```python
from build123d import *

# Parameters (mm, degrees)
BOSS_EXTRUDE1_DEPTH  = 557.5
SKETCH2_W            = 37.5
SKETCH2_H            = 40
BOSS_EXTRUDE2_DEPTH  = 340
BOSS_EXTRUDE3_DEPTH  = 1115
SKETCH4_W            = 120
SKETCH4_H            = 22
CUT_EXTRUDE1_DEPTH   = 754.951092578
FILLET1_R            = 6
SKETCH8_W            = 20
SKETCH8_H            = 10
CUT_EXTRUDE3_DEPTH   = 754.951092578
SKETCH9_W            = 25
SKETCH9_H            = 25
SKETCH9_R            = 5.25
BOSS_EXTRUDE6_DEPTH  = 20
CHAMFER1_SIZE        = 4
SKETCH10_W           = 1014
SKETCH10_H           = 110
BOSS_EXTRUDE7_DEPTH  = 15
BOSS_EXTRUDE8_DEPTH  = 507
BOSS_EXTRUDE9_DEPTH  = 5
BOSS_EXTRUDE10_START = -14
SKETCH13_W           = 70
SKETCH13_H           = 58
BOSS_EXTRUDE10_DEPTH = 45


with BuildPart() as part:
    # Sketch1 → Boss-Extrude1 (new, symmetric)
    with BuildSketch(Plane(origin=(0, 0, 0), x_dir=(0, 0, -1), z_dir=(1, 0, 0))):
        Polygon((0, 0), (0, 83), (40, 83), (40, 16), (20.823523748, 16), (15, 0), align=None)
    extrude(amount=BOSS_EXTRUDE1_DEPTH, both=True)

    # Sketch2 → Boss-Extrude2 (add)
    with BuildSketch(Plane(origin=(0, 83, 0), x_dir=(1, 0, 0), z_dir=(0, 1, 0))):
        with Locations((-534.75, 20)):
            Rectangle(SKETCH2_W, SKETCH2_H)
        with Locations((534.75, 20)):
            Rectangle(SKETCH2_W, SKETCH2_H)
    extrude(amount=BOSS_EXTRUDE2_DEPTH)

    # Sketch3 → Boss-Extrude3 (add)
    with BuildSketch(Plane(origin=(557.5, 0, 0), x_dir=(0, 0, -1), z_dir=(1, 0, 0))):
        Polygon((0, 423), (0, 506), (15, 506), (20.823523748, 490), (40, 490), (40, 423), align=None)
    extrude(amount=-BOSS_EXTRUDE3_DEPTH)

    # Sketch4 → Cut-Extrude1 (cut, through all)
    with BuildSketch(Plane.XY):
        with Locations((38.5, 11)):
            Rectangle(SKETCH4_W, SKETCH4_H)
    extrude(amount=-CUT_EXTRUDE1_DEPTH, mode=Mode.SUBTRACT)

    # Fillet1
    fillet1_edges = [part.edges().sort_by_distance(p)[0] for p in [
        (98.5, 22, -20),
        (-21.5, 22, -20),
    ]]
    fillet(fillet1_edges, radius=FILLET1_R)

    # Sketch8 → Cut-Extrude3 (cut, through all)
    with BuildSketch(Plane.XY):
        with Locations((-461.5, 501)):
            Rectangle(SKETCH8_W, SKETCH8_H)
        with Locations((-385.416666667, 501)):
            Rectangle(SKETCH8_W, SKETCH8_H)
        with Locations((-309.333333333, 501)):
            Rectangle(SKETCH8_W, SKETCH8_H)
        with Locations((-233.25, 501)):
            Rectangle(SKETCH8_W, SKETCH8_H)
        with Locations((-157.166666667, 501)):
            Rectangle(SKETCH8_W, SKETCH8_H)
        with Locations((-81.083333333, 501)):
            Rectangle(SKETCH8_W, SKETCH8_H)
        with Locations((-5, 501)):
            Rectangle(SKETCH8_W, SKETCH8_H)
        with Locations((71.083333333, 501)):
            Rectangle(SKETCH8_W, SKETCH8_H)
        with Locations((147.166666667, 501)):
            Rectangle(SKETCH8_W, SKETCH8_H)
        with Locations((223.25, 501)):
            Rectangle(SKETCH8_W, SKETCH8_H)
        with Locations((299.333333333, 501)):
            Rectangle(SKETCH8_W, SKETCH8_H)
        with Locations((375.416666667, 501)):
            Rectangle(SKETCH8_W, SKETCH8_H)
        with Locations((451.5, 501)):
            Rectangle(SKETCH8_W, SKETCH8_H)
    extrude(amount=-CUT_EXTRUDE3_DEPTH, mode=Mode.SUBTRACT)

    # Sketch9 → Boss-Extrude6 (add)
    with BuildSketch(Plane.XY):
        with Locations((0, 95.5)):
            Rectangle(SKETCH9_W, SKETCH9_H)
        with Locations((0, 95.5)):
            Circle(SKETCH9_R, mode=Mode.SUBTRACT)
    extrude(amount=-BOSS_EXTRUDE6_DEPTH)

    # Chamfer1
    chamfer1_edges = [part.edges().sort_by_distance(p)[0] for p in [
        (-12.5, 83, -10),
        (-12.5, 108, -10),
        (12.5, 108, -10),
        (12.5, 83, -10),
    ]]
    chamfer(chamfer1_edges, length=CHAMFER1_SIZE)

    # Sketch10 → Boss-Extrude7 (add)
    with BuildSketch(Plane(origin=(0, 0, -40), x_dir=(-1, 0, 0), z_dir=(0, 0, -1))):
        with Locations((0, 491)):
            Rectangle(SKETCH10_W, SKETCH10_H)
    extrude(amount=BOSS_EXTRUDE7_DEPTH)

    # Sketch11 → Boss-Extrude8 (add, symmetric)
    with BuildSketch(Plane(origin=(0, 0, 0), x_dir=(0, 0, -1), z_dir=(1, 0, 0))):
        Polygon((55, 536), (100, 536), (100, 496), (93.279404685, 496), (86, 516), (55, 516), align=None)
    extrude(amount=BOSS_EXTRUDE8_DEPTH, both=True)

    # Sketch12 → Boss-Extrude9 (add)
    with BuildSketch(Plane.XY.offset(-40)):
        with BuildLine():
            Line((-25, 546), (-25, 576))
            ThreePointArc((-25, 576), (0, 601), (25, 576))
            Line((25, 576), (25, 546))
            Line((25, 546), (-25, 546))
        make_face()
        with BuildLine():
            Line((-15, 556), (-15, 576))
            ThreePointArc((-15, 576), (0, 591), (15, 576))
            Line((15, 576), (15, 556))
            Line((15, 556), (-15, 556))
        make_face(mode=Mode.SUBTRACT)
    extrude(amount=-BOSS_EXTRUDE9_DEPTH)

    # Sketch13 → Boss-Extrude10 (add)
    with BuildSketch(Plane.XY.offset(BOSS_EXTRUDE10_START)):
        with Locations((-331, 394)):
            Rectangle(SKETCH13_W, SKETCH13_H)
    extrude(amount=-BOSS_EXTRUDE10_DEPTH)


solid = part.part
```
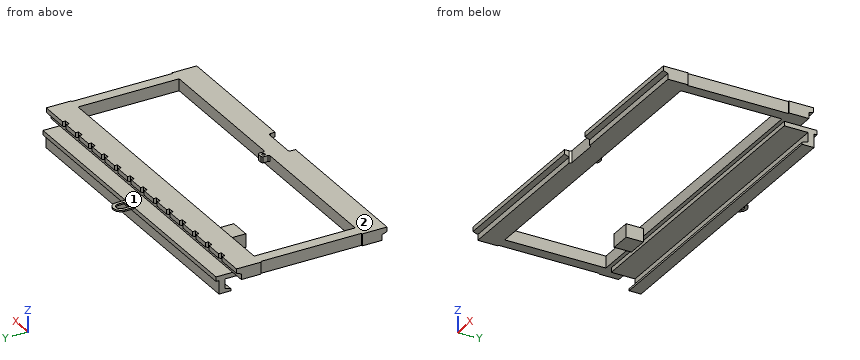
Could you check a few things on this model? Use its own coordinates, in mm. Face numbers are marked on the shaded views. Coordinates: 2 decimals unless noted, no trailing zeros. Order: outer loops, then holes, each group sorted by start corner. A loop starts at its lowest first (then second) coordinate and runs counter-clockwise, first axis right, second up. Notation, with made-up numbers: M -19.5,0 L 29.5,0 A21 ccw 29.5,26 Z; hole C 86,7 d3. An arc over 180 degrees is marked long. Use a Markdown table: item, result. Add a question column.
Q1. I want a section at A-A on x = 260. List the corners of the cut face in (y, z) for me, then the cut area to 3 significant figures.
Q2. If I drill on L1, parallel to Y at x = 0, z = -10.5; L2, parallel to X at y = 95, z = -11; L3, parallel to X at y = 142, z = -21.5, over which ranges is the centre line in solid material (lowest first)?
Q3. I'm going to push flat-ended pins straight in: pin 1 (4.5 mm diameter, centred on x = 249, z = -8.5, fed in from +Y); pin 2 (1 mm diameter, centred on x = 28, z = -85, fed in from -Y); pin 3 (1 mm diameter, centred on x = -51.5, y = 459, fed in from -Z). Where does each tip first touch, or does it pass through?
Q4. I want a section at D-D on y = 65.5. List the corners of the cut face in (x, z) for me, then the cut area to 3 significant figures.
Q5. I want a section at C-C on y = 469. List the corners of the cut face in (x, z) for me.
Q6. We'd pull the mould along Z, two halves only. Please class the marked faces 1 and 2: pulls with the +Z half, pulls with the -Z half, needs draft (parallel to the pull), parting line crosses it, or undercut.
Q7. I want a section at B-B on y = 234.5. List the corners of the cut face in (x, z) for me.
Checked values:
| question | item | result |
|---|---|---|
| 1 | outline | M 0,-15 L 16,-20.82 L 16,-40 L 83,-40 L 83,0 L 0,0 Z; M 423,-40 L 436,-40 L 436,-55 L 516,-55 L 516,-86 L 496,-93.28 L 496,-100 L 536,-100 L 536,-55 L 546,-55 L 546,-40 L 490,-40 L 490,-20.82 L 506,-15 L 506,0 L 423,0 Z |
| 1 | area | 8,690 mm² |
| 2 | L1 | 22 to 90.25, 100.75 to 108, 423 to 496 |
| 2 | L2 | -553.5 to -516, -12.5 to -5.23, 5.23 to 12.5, 516 to 553.5 |
| 2 | L3 | -553.5 to -516, 516 to 553.5 |
| 3 | pin 1 | y = 506 |
| 3 | pin 2 | y = 516 |
| 3 | pin 3 | z = -55 |
| 4 | outline | M -557.5,-40 L 557.5,-40 L 557.5,0 L -557.5,0 Z |
| 4 | area | 44,600 mm² |
| 5 | outline | M -557.5,-40 L -507,-40 L -507,-55 L 507,-55 L 507,-40 L 557.5,-40 L 557.5,0 L -557.5,0 Z |
| 6 | face 1 | undercut |
| 6 | face 2 | pulls with the +Z half |
| 7 | outline | M -553.5,-40 L -516,-40 L -516,0 L -553.5,0 Z; M 516,-40 L 553.5,-40 L 553.5,0 L 516,0 Z |
